```python
from build123d import *

# Parameters (mm, degrees)
SKETCH1_W                = 18
SKETCH1_H                = 39
SKETCH1_W_2              = 20
BOSS_EXTRUDE1_DEPTH      = 10
BOSS_EXTRUDE3_REACH      = 74.32
SKETCH3_R                = 7.5
SKETCH4_R                = 5
CUT_EXTRUDE1_DEPTH       = 68
CUT_EXTRUDE2_DEPTH       = 5
BOSS_EXTRUDE4_START      = 3
SKETCH6_R                = 8
SKETCH6_R_2              = 5
BOSS_EXTRUDE4_DEPTH      = 3
BOSS_EXTRUDE5_DEPTH      = 1
SKETCH8_W                = 48
SKETCH8_H                = 12
BOSS_EXTRUDE6_DEPTH      = 1
CHAMFER1_SIZE            = 1
CHAMFER1_OF_MIRROR2_SIZE = 1


with BuildPart() as part:
    # Sketch1 → Boss-Extrude1 (new, symmetric)
    with BuildSketch(Plane(origin=(0, 0, 0), x_dir=(1, 0, 0), z_dir=(0, 1, 0))):
        with BuildLine():
            Line((0, -22.5), (-58, -22.5))
            ThreePointArc((-58, -22.5), (-65.071067812, -19.571067812), (-68, -12.5))
            Line((-68, -12.5), (-68, 12.5))
            ThreePointArc((-68, 12.5), (-65.071067812, 19.571067812), (-58, 22.5))
            Line((-58, 22.5), (0, 22.5))
            Line((0, 22.5), (0, -22.5))
        make_face()
        with Locations((-12, 0)):
            Rectangle(SKETCH1_W, SKETCH1_H, mode=Mode.SUBTRACT)
        with BuildLine():
            Line((-65, -12.5), (-65, 12.5))
            ThreePointArc((-65, 12.5), (-62.949747468, 17.449747468), (-58, 19.5))
            Line((-58, 19.5), (-47, 19.5))
            Line((-47, 19.5), (-47, -19.5))
            Line((-47, -19.5), (-58, -19.5))
            ThreePointArc((-58, -19.5), (-62.949747468, -17.449747468), (-65, -12.5))
        make_face(mode=Mode.SUBTRACT)
        with Locations((-34, 0)):
            Rectangle(SKETCH1_W_2, SKETCH1_H, mode=Mode.SUBTRACT)
    extrude(amount=BOSS_EXTRUDE1_DEPTH, both=True)

    # Boss-Extrude3: up to this face of the body (flat: up to its plane)
    boss_extrude3_end = Plane(part.part.faces().sort_by_distance((-65, 0, 0))[0])
    # Sketch3 → Boss-Extrude3 (add, up to the picked face)
    with BuildSketch(Plane(origin=(0, 0, 0), x_dir=(0, 0, -1), z_dir=(1, 0, 0)), mode=Mode.PRIVATE) as boss_extrude3_sk1:
        Circle(SKETCH3_R)
    boss_extrude3_tool1 = split(extrude(boss_extrude3_sk1.sketch, amount=-BOSS_EXTRUDE3_REACH, mode=Mode.PRIVATE), bisect_by=boss_extrude3_end, keep=Keep.BOTH, mode=Mode.PRIVATE)
    add(boss_extrude3_tool1.solids().sort_by(Axis((0, 0, 0), (-1, 0, 0)))[0])

    # Sketch4 → Cut-Extrude1 (cut)
    with BuildSketch(Plane(origin=(0, 0, 0), x_dir=(0, 0, -1), z_dir=(1, 0, 0))):
        Circle(SKETCH4_R)
    extrude(amount=-CUT_EXTRUDE1_DEPTH, mode=Mode.SUBTRACT)

    # Sketch5 → Cut-Extrude2 (cut)
    with BuildSketch(Plane.ZY.offset(68)):
        Polygon((3.464101615, 6), (-3.464101615, 6), (-6.92820323, 0), (-3.464101615, -6), (3.464101615, -6), (6.92820323, 0), align=None)
    extrude(amount=-CUT_EXTRUDE2_DEPTH, mode=Mode.SUBTRACT)

    # Sketch6 → Boss-Extrude4 (add)
    with BuildSketch(Plane(origin=(0, 0, 0), x_dir=(0, 0, -1), z_dir=(1, 0, 0)).offset(BOSS_EXTRUDE4_START)):
        with Locations(Location((0, 0, 0), (0, 0, 180))):
            Circle(SKETCH6_R)
        Circle(SKETCH6_R_2, mode=Mode.SUBTRACT)
    extrude(amount=-BOSS_EXTRUDE4_DEPTH)

    # Sketch7 → Boss-Extrude5 (add)
    with BuildSketch(Plane(origin=(0, 10, 0), x_dir=(1, 0, 0), z_dir=(0, 1, 0))):
        with BuildLine():
            Line((-16.5, 19.5), (-28.5, 19.5))
            ThreePointArc((-28.5, 19.5), (-30, 21), (-28.5, 22.5))
            Line((-28.5, 22.5), (-16.5, 22.5))
            ThreePointArc((-16.5, 22.5), (-15, 21), (-16.5, 19.5))
        make_face()
        with BuildLine():
            Line((-51.5, 22.5), (-39.5, 22.5))
            ThreePointArc((-39.5, 22.5), (-38, 21), (-39.5, 19.5))
            Line((-39.5, 19.5), (-51.5, 19.5))
            ThreePointArc((-51.5, 19.5), (-53, 21), (-51.5, 22.5))
        make_face()
        with BuildLine():
            Line((-16.5, -19.5), (-28.5, -19.5))
            ThreePointArc((-28.5, -19.5), (-30, -21), (-28.5, -22.5))
            Line((-28.5, -22.5), (-16.5, -22.5))
            ThreePointArc((-16.5, -22.5), (-15, -21), (-16.5, -19.5))
        make_face()
        with BuildLine():
            Line((-51.5, -22.5), (-39.5, -22.5))
            ThreePointArc((-39.5, -22.5), (-38, -21), (-39.5, -19.5))
            Line((-39.5, -19.5), (-51.5, -19.5))
            ThreePointArc((-51.5, -19.5), (-53, -21), (-51.5, -22.5))
        make_face()
        with BuildLine():
            Line((-68, -6), (-68, 6))
            ThreePointArc((-68, 6), (-66.5, 7.5), (-65, 6))
            Line((-65, 6), (-65, -6))
            ThreePointArc((-65, -6), (-66.5, -7.5), (-68, -6))
        make_face()
        with BuildLine():
            Line((-24, -6), (-24, 6))
            ThreePointArc((-24, 6), (-22.5, 7.5), (-21, 6))
            Line((-21, 6), (-21, -6))
            ThreePointArc((-21, -6), (-22.5, -7.5), (-24, -6))
        make_face()
        with BuildLine():
            Line((-47, -6), (-47, 6))
            ThreePointArc((-47, 6), (-45.5, 7.5), (-44, 6))
            Line((-44, 6), (-44, -6))
            ThreePointArc((-44, -6), (-45.5, -7.5), (-47, -6))
        make_face()
        with BuildLine():
            Line((-3, -6), (-3, 6))
            ThreePointArc((-3, 6), (-1.5, 7.5), (0, 6))
            Line((0, 6), (0, -6))
            ThreePointArc((0, -6), (-1.5, -7.5), (-3, -6))
        make_face()
    boss_extrude5 = extrude(amount=BOSS_EXTRUDE5_DEPTH)

    # Mirror1: Boss-Extrude5 across plane
    add(boss_extrude5.mirror(Plane.ZX))

    # Sketch8 → Boss-Extrude6 (add)
    with BuildSketch(Plane.XY.offset(22.5)):
        with Locations((-29, 0)):
            Rectangle(SKETCH8_W, SKETCH8_H)
    boss_extrude6 = extrude(amount=BOSS_EXTRUDE6_DEPTH)

    # Chamfer1
    chamfer1_edges = [part.edges().sort_by_distance(p)[0] for p in [
        (-53, 0, 23.5),
        (-29, -6, 23.5),
        (-5, 0, 23.5),
        (-29, 6, 23.5),
    ]]
    chamfer(chamfer1_edges, length=CHAMFER1_SIZE - 0.0001)  # a hair under: the kernel refuses the full size

    # Mirror2: Boss-Extrude6 across plane
    add(boss_extrude6.mirror(Plane.XY))

    # Chamfer1 of Mirror2
    chamfer1_of_mirror2_edges = [part.edges().sort_by_distance(p)[0] for p in [
        (-53, 0, -23.5),
        (-29, -6, -23.5),
        (-5, 0, -23.5),
        (-29, 6, -23.5),
    ]]
    chamfer(chamfer1_of_mirror2_edges, length=CHAMFER1_OF_MIRROR2_SIZE - 0.0001)  # a hair under: the kernel refuses the full size


solid = part.part
```
Input: part model. Units: mm. Frame: model coordinates. A direction names the side the tool comes from. Give positions to 0.01 mm unless a question says otherwise; leave off trailing zeros. Return JSON: item names as keys, results as strings.
1) Mould query, pull axis X, two halves, no side actions, for faces 6 (the face through (-68, 3, 6)), 7 (the face through (-66.5, 10.5, -7.5)), 8 (the face through (-65.535, -3.042, 5.172)). Classes: released by +X, released by -X, zero draft, split by the parting line, or undercut.
Taken from the geometry:
{"face 6": "released by -X", "face 7": "undercut", "face 8": "zero draft"}
2) Access query for faces 1 (the face through (-62.9, 0.1, 17.5)), 2 (the face through (-30, -10.5, 21)), 3 (the face through (-53, 10.5, -21)), 4 (the face through (-1, -11, 0)), 5 (the face through (-45.5, 10.5, -7.5)). Directions: +Z, -Z, +X, -X, +Y, -Y. A direction counts if a zero-diameter tool reaches every point of the face in a straight line with its end or side. Return the directions, or none.
Taken from the geometry:
{"face 1": "+Y, -Y", "face 2": "-Y", "face 3": "-X, +Y", "face 4": "+Z, -Z, +X, -X, -Y", "face 5": "+Y"}
3) Contact query for flat-ended pins moving along their axis: pin 1 (6 mm diameter, centred on x = -57, y = -5.5, fed in from +Z); pin 2 (3.5 mm diameter, centred on x = -46, z = -13.5, fed in from +Y); pin 3 (1.5 mm diameter, centred on y = -8.5, z = 6, fed in from +X). Output: stop coordinate, or through.
Taken from the geometry:
{"pin 1": "stops at z = 22.5", "pin 2": "stops at y = 10", "pin 3": "stops at x = 0"}
4) Section query A-A on x = -10. Count the separate pieces of the cut face and the enclosed holes in it, and give its area (3 significant figures).
Taken from the geometry:
{"separate pieces": "3", "enclosed holes": "1", "area": "240 mm2"}
5) Line query: L1, parallel to X at y = 7, z = 10.5; L2, parallel to Z at x = -42.5, y = 8.5; L3, parallel to Y at x = -46.5, z = 0. Output: solid intervals per line, ascending. Write a range as [from, to].
Taken from the geometry:
{"L1": "x = [-68, -65], [-47, -44], [-24, -21], [-3, 0]", "L2": "z = [-22.5, -19.5], [19.5, 22.5]", "L3": "y = [-11, -5], [5, 11]"}
